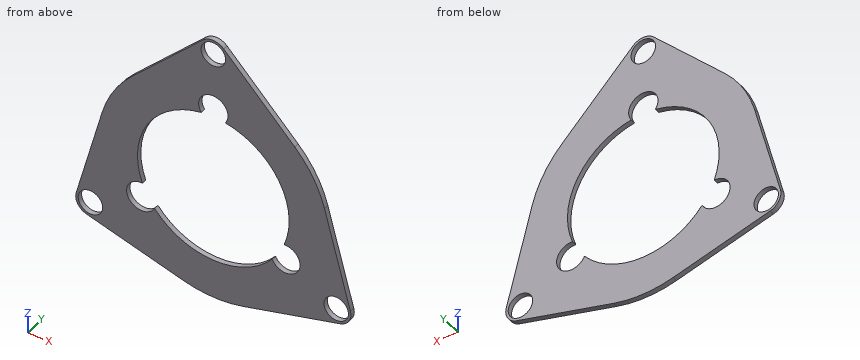
```python
from build123d import *

# Parameters (mm, degrees)
ESQUISSE1_R      = 1.25
EXTRUSION1_DEPTH = 0.5


with BuildPart() as part:
    # Esquisse1 → Extrusion1 (new body)
    with BuildSketch(Plane(origin=(0, 0, 0), x_dir=(1, 0, 0), z_dir=(0, 1, 0))):
        with BuildLine():
            Line((-11.352572917, -3.041912745), (-14.006257094, 6.861771432))
            ThreePointArc((-14.006257094, 6.861771432), (-13.856406461, 8), (-12.945596923, 8.698888739))
            Line((-12.945596923, 8.698888739), (-3.041912745, 11.352572917))
            ThreePointArc((-3.041912745, 11.352572917), (0, 11.753048327), (3.041912745, 11.352572917))
            Line((3.041912745, 11.352572917), (12.945596923, 8.698888739))
            ThreePointArc((12.945596923, 8.698888739), (13.856406461, 8), (14.006257094, 6.861771432))
            Line((14.006257094, 6.861771432), (11.352572917, -3.041912745))
            ThreePointArc((11.352572917, -3.041912745), (10.178438423, -5.876524164), (8.310660172, -8.310660172))
            Line((8.310660172, -8.310660172), (1.060660172, -15.560660172))
            ThreePointArc((1.060660172, -15.560660172), (0, -16), (-1.060660172, -15.560660172))
            Line((-1.060660172, -15.560660172), (-8.310660172, -8.310660172))
            ThreePointArc((-8.310660172, -8.310660172), (-10.178438423, -5.876524164), (-11.352572917, -3.041912745))
        make_face()
        with Locations((-12.557368355, 7.25)):
            Circle(ESQUISSE1_R, mode=Mode.SUBTRACT)
        with Locations((12.557368355, 7.25)):
            Circle(ESQUISSE1_R, mode=Mode.SUBTRACT)
        with Locations((0, -14.5)):
            Circle(ESQUISSE1_R, mode=Mode.SUBTRACT)
        with BuildLine():
            ThreePointArc((-7.243944164, 2.754591249), (-8.660254038, 5), (-6.007518081, 4.896144045))
            ThreePointArc((-6.007518081, 4.896144045), (0, 7.75), (6.007518081, 4.896144045))
            ThreePointArc((6.007518081, 4.896144045), (8.660254038, 5), (7.243944164, 2.754591249))
            ThreePointArc((7.243944164, 2.754591249), (6.711696879, -3.875), (1.236426083, -7.650735294))
            ThreePointArc((1.236426083, -7.650735294), (0, -10), (-1.236426083, -7.650735294))
            ThreePointArc((-1.236426083, -7.650735294), (-6.711696879, -3.875), (-7.243944164, 2.754591249))
        make_face(mode=Mode.SUBTRACT)
    extrude(amount=EXTRUSION1_DEPTH)


solid = part.part
```
Part model, mm, in its own coordinate system. Coordinates: 2 decimals unless noted, no trailing zeros. Write each loop counter-clockwise with the first axis right and the second up, starting at its lowest first coordinate (ties: lowest second). Pieces come first, ordered by that corner, then holes.
Item 1: Slice it at B-B (z = -4.25). Write the cut outline in (x, y), and give its area (3 significant figures).
Item 2: Slice it at C-C (y = 0.2). Write the cut outline in (x, z).
Item 3: Slice it at A-A (x = -4.5). Write the cut outline in (y, z), and give its area (3 significant figures).
Item 4: Slice it at D-D (z = -7.25). Write the cut outline in (x, y).
Item 5: Probe line 1 (Z direction, x = 1, y = 0.45); line 2 (Z direction, x = -0.75, y = 0.3); line 3 (X direction, y = 0.25, z = -6.25). List the from-to ranges inside material, lowest first.
Item 6: Pin check, flat tips, straight feed: pin 1 (2.5 mm diameter, centred on x = 7.36, z = -4.25, fed in from +Y); pin 2 (3 mm diameter, centred on x = -12.56, z = -7.25, fed in from -Y). Stop position of each tip, or through.
Results found:
1. outline: (-13.31, 0) - (-8.86, 0) - (-8.86, 0.5) - (-13.31, 0.5) - close; (8.86, 0) - (13.31, 0) - (13.31, 0.5) - (8.86, 0.5) - close
1. area: 4.45 mm2
2. outline: (-14.01, -6.86) arc R1.5 ccw to (-12.95, -8.7) - (-3.04, -11.35) arc R11.75 ccw to (3.04, -11.35) - (12.95, -8.7) arc R1.5 ccw to (14.01, -6.86) - (11.35, 3.04) arc R11.75 ccw to (8.31, 8.31) - (1.06, 15.56) arc R1.5 ccw to (-1.06, 15.56) - (-8.31, 8.31) arc R11.75 ccw to (-11.35, 3.04) - close; hole circle Ø2.5 at (-12.56, -7.25); hole (-7.24, -2.75) arc R1.5 ccw (long way) to (-6.01, -4.9) arc R7.75 ccw to (6.01, -4.9) arc R1.5 ccw (long way) to (7.24, -2.75) arc R7.75 ccw to (1.24, 7.65) arc R1.5 ccw (long way) to (-1.24, 7.65) arc R7.75 ccw to start; hole circle Ø2.5 at (0, 14.5); hole circle Ø2.5 at (12.56, -7.25)
3. outline: (0, -10.96) - (0.5, -10.96) - (0.5, -6.31) - (0, -6.31) - close; (0, 6.31) - (0.5, 6.31) - (0.5, 12.12) - (0, 12.12) - close
3. area: 5.23 mm2
4. outline: (-14.06, 0) - (-13.81, 0) - (-13.81, 0.5) - (-14.06, 0.5) - close; (-11.31, 0) - (-2.74, 0) - (-2.74, 0.5) - (-11.31, 0.5) - close; (2.74, 0) - (11.31, 0) - (11.31, 0.5) - (2.74, 0.5) - close; (13.81, 0) - (14.06, 0) - (14.06, 0.5) - (13.81, 0.5) - close
5. line 1: z = -11.71 to -7.69, 9.62 to 13.75, 15.25 to 15.62
5. line 2: z = -11.73 to -7.71, 9.8 to 13.5, 15.5 to 15.8
5. line 3: x = -13.84 to -13.31, -11.81 to -4.58, 4.58 to 11.81, 13.31 to 13.84
6. pin 1: passes through
6. pin 2: stops at y = 0
